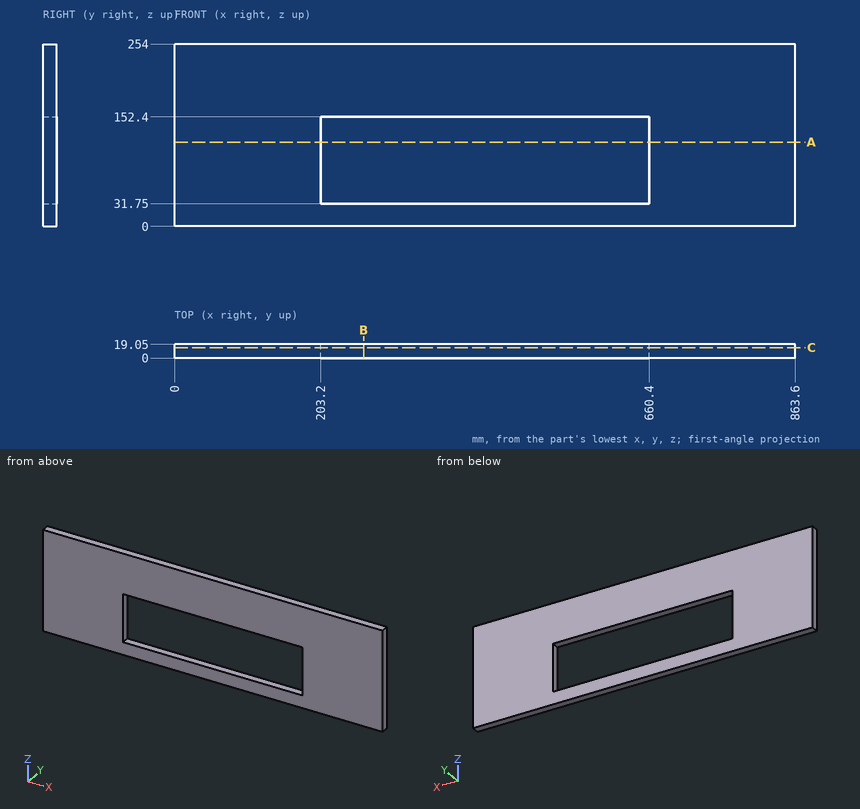
Input: dimensioned drawing with shaded views. Units: mm. Origin: part minimum x, y, z. Round coordinates to 2 decimals unless told otherwise and drop trailing zeros. Write each loop counter-clockwise with the first axis right and the second up, starting at its lowest first coordinate (ties: lowest second). Pieces come first, ordered by that corner, then holes. Notation, with made-up numbers: (9.5, 37.5) -> (52.5, 37.5) arc R7 ccw to (52.5, 43.5) -> close; hole circle Ø11 at (-4.75, -25). An arc over 180 degrees is marked (long way). Use CSV: the item, a comma, the result in double quotes. Start each with the question number.
Q1. Section B-B (x = 263). Return loops of the section in (y, z), plus the area to 3 significant figures.
Q2. Line query: L1, parallel to X at y = 17.75, z = 89.5; L2, parallel to Z at x = 527.5, y = 11.75. Output: solid intervals per line, ascending.
Q3. Section A-A (z = 117.5). Return loops of the section in (x, y), plus the area to 3 significant figures.
Q4. Section C-C (y = 14.5). Return loops of the section in (x, z).
Result sheet:
1,outline,"(0, 0) -> (19.05, 0) -> (19.05, 31.75) -> (0, 31.75) -> close; (0, 152.4) -> (19.05, 152.4) -> (19.05, 254) -> (0, 254) -> close"
1,area,"2,540 mm²"
2,L1,"0 to 203.2, 660.4 to 863.6"
2,L2,"0 to 31.75, 152.4 to 254"
3,outline,"(0, 0) -> (203.2, 0) -> (203.2, 19.05) -> (0, 19.05) -> close; (660.4, 0) -> (863.6, 0) -> (863.6, 19.05) -> (660.4, 19.05) -> close"
3,area,"7,740 mm²"
4,outline,"(0, 0) -> (863.6, 0) -> (863.6, 254) -> (0, 254) -> close; hole (203.2, 31.75) -> (660.4, 31.75) -> (660.4, 152.4) -> (203.2, 152.4) -> close"
